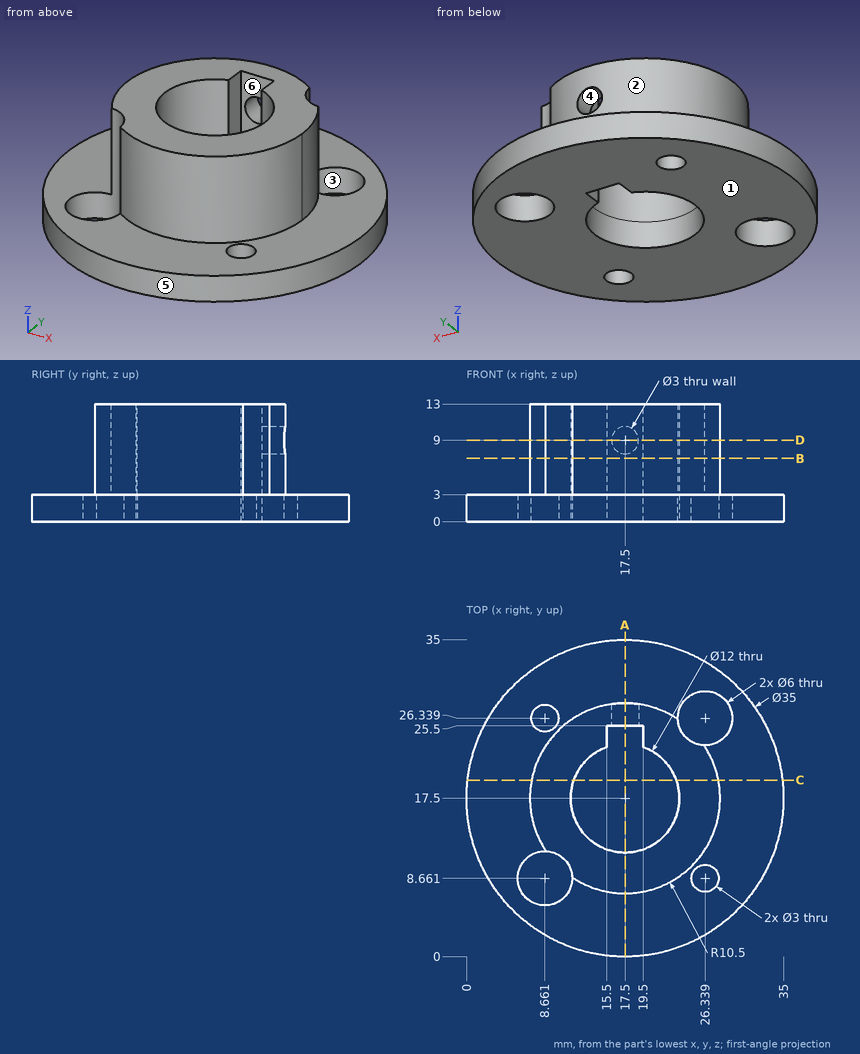
Study the drawing (mm; zero at the part's minimum x, y, z) and answer. A direction names the side the tool comes from. Round coordinates to 2 decimals unless told otherwise and drop trailing zeros. Write each loop counter-clockwise with the first axis right and the second up, starting at its lowest first coordinate (ties: lowest second). Pieces come first, ordered by that corner, then holes.
Q1. The mould has two halves that part along Y. Classify the marked faces 3, 4, 5 and 6: released by +Y, released by -Y, zero draft, split by the parting line, or undercut.
Values:
face 3: undercut
face 4: zero draft
face 5: split by the parting line
face 6: undercut
Q2. Find section C-C on y = 19.5. Determine the outline of the cut face in (x, z) (1 decimal).
Values:
outline: (0.1, 0) - (11.8, 0) - (11.8, 13) - (7.2, 13) - (7.2, 3) - (0.1, 3) - close; (23.2, 0) - (34.9, 0) - (34.9, 3) - (27.8, 3) - (27.8, 13) - (23.2, 13) - close
Q3. Find section A-A on x = 17.5. Determine the outline of the cut face in (y, z), and give its area (4 significant figures).
Values:
outline: (0, 0) - (11.5, 0) - (11.5, 13) - (7, 13) - (7, 3) - (0, 3) - close; (25.5, 0) - (35, 0) - (35, 3) - (28, 3) - (28, 7.5) - (25.5, 7.5) - close; (25.5, 10.5) - (28, 10.5) - (28, 13) - (25.5, 13) - close
area: 125.5 mm2
Q4. Find section B-B on z = 7. Determine the outline of the cut face in (x, y).
Values:
outline: (8.77, 11.66) arc R3 cw to (11.66, 8.77) arc R10.5 ccw to (26.23, 23.34) arc R3 cw to (23.34, 26.23) arc R10.5 ccw to start; hole (15.5, 23.16) arc R6 ccw (long way) to (19.5, 23.16) - (19.5, 25.5) - (15.5, 25.5) - close
Q5. Straight lines are drawn through the part: line 1 (Y direction, x = 25.5, z = 0.75) (1 decimal); line 2 (Y direction, x = 17.5, z = 6.75); line 3 (Z direction, x = 2.5, y = 10.5). For each, find the intervals that lie inside material, in ascending order.
Values:
line 1: y = 1.9 to 7.4, 9.9 to 23.5, 29.2 to 33.1
line 2: y = 7 to 11.5, 25.5 to 28
line 3: z = 0 to 3
Q6. Flat-ended cylindrical pins translate along their axes: P1, Ø4, axis at x = 17.5, z = 9, coming from the +Y side; P2, Ø1.5, axis at x = 14.5, z = 9, coming from the +Y side; P3, Ø1, axis at x = 28.5, y = 28, coming from the +Z side; P4, Ø11, axis at x = 17.5, y = 17.5, coming from the +Z side. Find the tip coordinate at first contact, or state that the pin passes through.
Values:
P1: stops at y = 28
P2: stops at y = 27.76
P3: stops at z = 3
P4: passes through
Q7. Find section D-D on z = 9. Determine the outline of the cut face in (x, y).
Values:
outline: (8.77, 11.66) arc R3 cw to (11.66, 8.77) arc R10.5 ccw to (26.23, 23.34) arc R3 cw to (23.34, 26.23) arc R10.5 ccw to (19, 27.89) - (19, 25.5) - (19.5, 25.5) - (19.5, 23.16) arc R6 cw (long way) to (15.5, 23.16) - (15.5, 25.5) - (16, 25.5) - (16, 27.89) arc R10.5 ccw to start
Q8. A tool of negligible diameter and unlimited length cuts with its end or side. For the marked faces 1 and 2, from which of +Z, -Z, +X, -X, +Y, -Y can it reach the whole face along a straight path? Write none if from no direction.
Values:
face 1: -Z, +X, -X, +Y, -Y
face 2: +Z
